Print and shaded views of the part. All mm, measured from the part's lowest x, y and z. A direction names the side the tool comes from. Round coordinates to 2 decimals unless told otherwise and drop trailing zeros. Write each loop counter-clockwise with the first axis right and the second up, starting at its lowest first coordinate (ties: lowest second). Pieces come first, ordered by that corner, then holes. Notation, with made-up numbers: (21, 67.5) - (58, 67.5) arc R6 ccw to (58, 74.5) - close; hole circle Ø2 at (13.5, -7). An arc over 180 degrees is marked (long way). Put each result on its own line as item: value. Start each with the question number.
Item 1: Pin check, flat tips, straight feed: pin 1 Ø1.5 at (x, z) = (2.5, 1.5) entering from -Y; pin 2 Ø1.5 at (y, z) = (1, 1.5) entering from +X; pin 3 Ø1 at (y, z) = (13.5, 2) entering from -X. Stop position of each tip, or through.
Item 2: Cut at C-C (z = 0.6). Give the cut face in (x, y), and give its area (3 significant figures).
Item 3: Mould opens along Y. For the marked faces 1, 2, 3 and 4 say: released by +Y, released by -Y, zero draft, split by the parting line, or undercut.
Item 4: Cut at A-A (x = 27). Give the cut face in (y, z), and give its area (3 significant figures).
Item 5: Cut at B-B (y = 7.25). Give the cut face in (x, z).
Item 6: 3-axis set-ups, long thin cutter, end or side, ignore diameter. For the marked faces 5 and 6: which of +Z, -Z, +X, -X, +Y, -Y reach the whole face in a straight line?
Item 7: Drill centre lines: line 1 (Y direction, x = 22, z = 0.4); line 2 (X direction, y = 2.5, z = 0.85); line 3 (X direction, y = 6.5, z = 2.05). Where is each one in solid material? Low to high. Write a range as from..to.
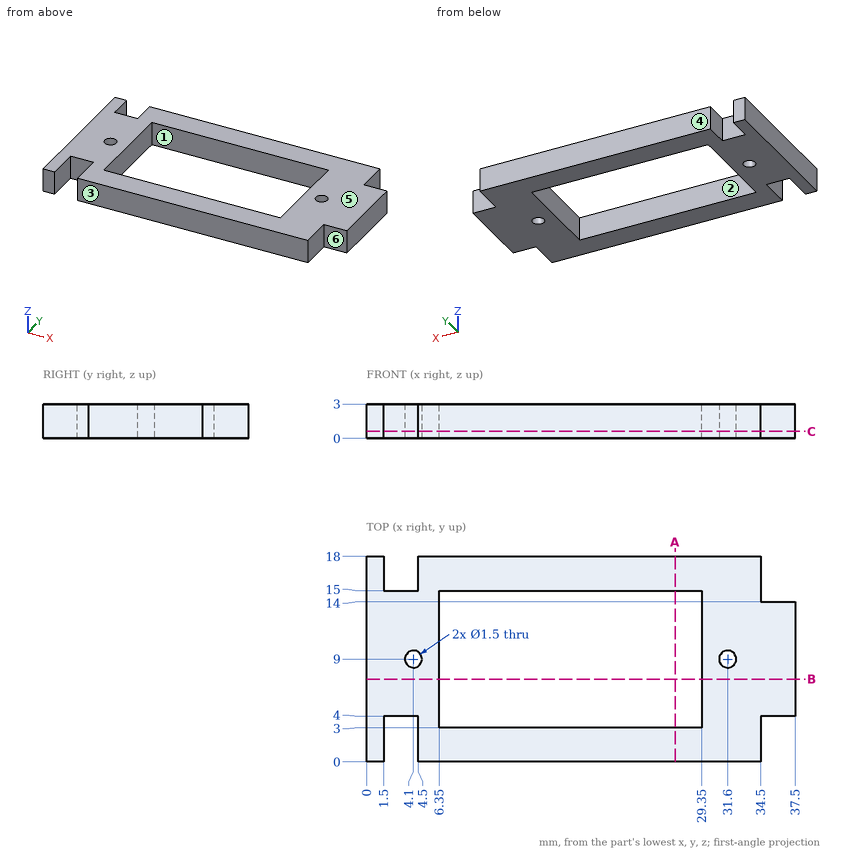
Output values:
1. pin 1: y = 4
1. pin 2: x = 34.5
1. pin 3: x = 0
2. outline: (0, 0) - (1.5, 0) - (1.5, 4) - (4.5, 4) - (4.5, 0) - (34.5, 0) - (34.5, 4) - (37.5, 4) - (37.5, 14) - (34.5, 14) - (34.5, 18) - (4.5, 18) - (4.5, 15) - (1.5, 15) - (1.5, 18) - (0, 18) - close; hole circle Ø1.5 at (4.1, 9); hole (6.35, 3) - (29.35, 3) - (29.35, 15) - (6.35, 15) - close; hole circle Ø1.5 at (31.6, 9)
2. area: 350 mm2
3. face 1: undercut
3. face 2: undercut
3. face 3: released by -Y
3. face 4: released by +Y
4. outline: (0, 0) - (3, 0) - (3, 3) - (0, 3) - close; (15, 0) - (18, 0) - (18, 3) - (15, 3) - close
4. area: 18.0 mm2
5. outline: (0, 0) - (6.35, 0) - (6.35, 3) - (0, 3) - close; (29.35, 0) - (37.5, 0) - (37.5, 3) - (29.35, 3) - close
6. face 5: +Z, +X, -X, +Y, -Y
6. face 6: +Z, -Z, +X, -Y
7. line 1: 0..3, 15..18
7. line 2: 0..1.5, 4.5..34.5
7. line 3: 0..6.35, 29.35..37.5
